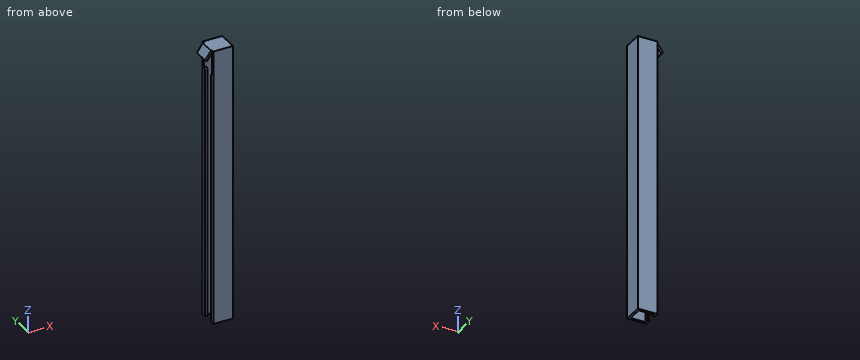
```python
from build123d import *

# Parameters (mm, degrees)
SKETCH1_W           = 16.6
SKETCH1_H           = 235
BOSS_EXTRUDE1_DEPTH = 2
SKETCH1_6_W         = 2
SKETCH1_6_H         = 214
BOSS_EXTRUDE3_DEPTH = 12.6
SKETCH3_W           = 16.6
SKETCH3_H           = 235
BOSS_EXTRUDE4_DEPTH = 2
SKETCH4_W           = 214
SKETCH4_H           = 8.6
CUT_EXTRUDE1_DEPTH  = 4
CUT_EXTRUDE2_DEPTH  = 4


with BuildPart() as part:
    # Sketch1 → Boss-Extrude1 (new body)
    with BuildSketch(Plane(origin=(0, 0, 0), x_dir=(1, 0, 0), z_dir=(0, 1, 0))):
        with Locations((8.3, 115.5)):
            Rectangle(SKETCH1_W, SKETCH1_H)
    extrude(amount=-BOSS_EXTRUDE1_DEPTH)

    # Sketch1<6> → Boss-Extrude3 (add)
    with BuildSketch(Plane(origin=(0, 0, 0), x_dir=(1, 0, 0), z_dir=(0, 1, 0))):
        with BuildLine():
            Line((-1.045606528, -2), (16.6, -2))
            Line((16.6, -2), (16.6, 233))
            Line((16.6, 233), (14.6, 233))
            Line((14.6, 233), (14.6, 14.47143967))
            ThreePointArc((14.6, 14.47143967), (10.315894346, 4.193033104), (0, 0))
            Line((0, 0), (-4.280197972, 6.15872595))
            Line((-4.280197972, 6.15872595), (-5.922524892, 5.017339824))
            Line((-5.922524892, 5.017339824), (-1.045606528, -2))
        make_face()
        with Locations((1, 126)):
            Rectangle(SKETCH1_6_W, SKETCH1_6_H)
    extrude(amount=BOSS_EXTRUDE3_DEPTH)

    # Sketch3 → Boss-Extrude4 (add)
    with BuildSketch(Plane(origin=(0, 12.6, 0), x_dir=(1, 0, 0), z_dir=(0, 1, 0))):
        with Locations((8.3, 115.5)):
            Rectangle(SKETCH3_W, SKETCH3_H)
    extrude(amount=BOSS_EXTRUDE4_DEPTH)

    # Sketch4 → Cut-Extrude1 (cut)
    with BuildSketch(Plane.ZY):
        with Locations((-126, 6.3)):
            Rectangle(SKETCH4_W, SKETCH4_H)
    extrude(amount=-CUT_EXTRUDE1_DEPTH, mode=Mode.SUBTRACT)

    # Sketch6 → Cut-Extrude2 (cut)
    with BuildSketch(Plane.ZY):
        with BuildLine():
            ThreePointArc((-20.999, 2), (-19.585493544, 1.414506456), (-19, 0.001))
            Line((-19, 0.001), (-19, 2))
            Line((-19, 2), (-20.999, 2))
        make_face()
        with BuildLine():
            Line((-19, 10.6), (-19, 12.599))
            ThreePointArc((-19, 12.599), (-19.585493544, 11.185493544), (-20.999, 10.6))
            Line((-20.999, 10.6), (-19, 10.6))
        make_face()
    extrude(amount=-CUT_EXTRUDE2_DEPTH, mode=Mode.SUBTRACT)


solid = part.part
```
Model file for the job. Use its own axes, mm. Coordinates: 2 decimals unless noted, no trailing zeros. Loops run counter-clockwise (first coordinate to the right, second up) from the corner with the lowest first, then second, coordinate; pieces in that order, holes last. Notation, with made-up numbers: (-22, 69.5) -> (10, 69.5) arc R22 ccw to (10, 92.5) -> close; hole circle Ø7 at (21, 11). An arc over 180 degrees is marked (long way). Answer as a JSON object with one key per item and string values.
Q1. Cut at A-A (y = 4.5). List the corners of the cut face in (x, z), and give its area (3 significant figures).
Report:
{"outline": "(-5.92, -5.02) -> (-4.28, -6.16) -> (0, 0) arc R14.47 cw to (14.6, -14.47) -> (14.6, -233) -> (16.6, -233) -> (16.6, 2) -> (-1.05, 2) -> close", "area": "561 mm2"}
Q2. Probe probe 1 along X at (y, z) = (11.5, -53); probe 2 along Y at (x, z) = (6, -169); probe 3 along X at (y, z) = (-1, -34). List the from-to ranges inside material, lowest first.
Report:
{"probe 1": "x = 0 to 2, 14.6 to 16.6", "probe 2": "y = -2 to 0, 12.6 to 14.6", "probe 3": "x = 0 to 16.6"}
Q3. Cut at B-B (z = -165.5). List the corners of the cut face in (x, y).
Report:
{"outline": "(0, -2) -> (16.6, -2) -> (16.6, 14.6) -> (0, 14.6) -> (0, 10.6) -> (2, 10.6) -> (2, 12.6) -> (14.6, 12.6) -> (14.6, 0) -> (2, 0) -> (2, 2) -> (0, 2) -> close"}
Q4. Cut at C-C (x = 9.25). List the corners of the cut face in (y, z), and give its area (3 significant figures).
Report:
{"outline": "(-2, -233) -> (0, -233) -> (0, -3.24) -> (12.6, -3.24) -> (12.6, -233) -> (14.6, -233) -> (14.6, 2) -> (-2, 2) -> close", "area": "1,010 mm2"}
Q5. Flat gauge pins, fed straight in: P1, Ø4, axis at x = -0.5, y = 4, coming from the -Z side; P2, Ø1.2, axis at y = -1, z = -145, coming from the -X side; P3, Ø4, axis at x = -3.5, z = -25.5, coming from the -Y side; P4, Ø1.8, axis at x = -4, z = -1, coming from the +Y side. Where does each tip first touch, or does it go through?
Report:
{"P1": "stops at z = -3.6", "P2": "stops at x = 0", "P3": "passes through", "P4": "stops at y = 12.6"}
